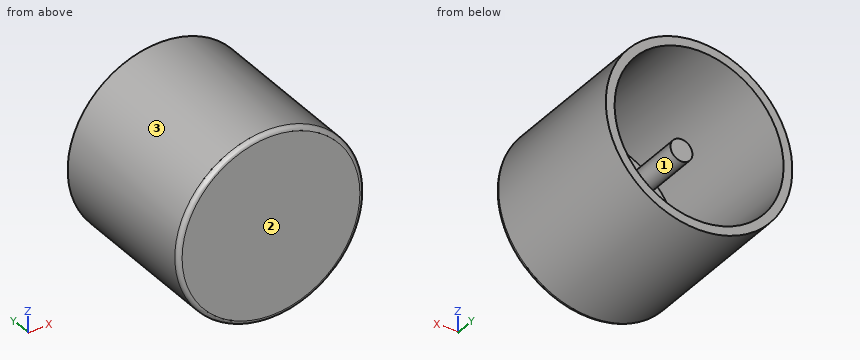
```python
from build123d import *

# Parameters (mm, degrees)
SKETCH1_R           = 53.975
BOSS_EXTRUDE1_DEPTH = 95.25
SHELL1_T            = -5.08
SKETCH2_R           = 6.35
BOSS_EXTRUDE2_DEPTH = 74.93
FILLET1_R           = 2.54


with BuildPart() as part:
    # Sketch1 → Boss-Extrude1 (new body)
    with BuildSketch(Plane(origin=(0, 0, 0), x_dir=(1, 0, 0), z_dir=(0, 1, 0))):
        with Locations(Location((0, 0, 0), (0, 0, 270))):
            Circle(SKETCH1_R)
    extrude(amount=BOSS_EXTRUDE1_DEPTH)

    # Shell1
    shell1_openings = [part.faces().sort_by_distance(p)[0] for p in [
        (0, 95.25, 0),
    ]]
    offset(amount=SHELL1_T, openings=shell1_openings, kind=Kind.INTERSECTION)

    # Sketch2 → Boss-Extrude2 (add)
    with BuildSketch(Plane(origin=(0, 5.08, 0), x_dir=(1, 0, 0), z_dir=(0, 1, 0))):
        with Locations(Location((0, 0, 0), (0, 0, 270))):
            Circle(SKETCH2_R)
    extrude(amount=BOSS_EXTRUDE2_DEPTH)

    # Fillet1
    fillet1_edges = [part.edges().sort_by_distance(p)[0] for p in [
        (0, 0, -53.975),
    ]]
    fillet(fillet1_edges, radius=FILLET1_R)


solid = part.part
```
Model file for the job. Use its own axes, mm. Face numbers are marked on the shaded views. Give positions to 0.01 mm unless a question says otherwise; leave off trailing zeros. Write each loop counter-clockwise with the first axis right and the second up, starting at its lowest first coordinate (ties: lowest second). Pieces come first, ordered by that corner, then holes. Notation, with made-up numbers: M -16,38 L 13,38 A9 cw 13,48 Z; hole C 74,48 d5. An arc over 180 degrees is marked long. Use a Markdown table: item, result.
1) Cut at C-C (z = 0). List the corners of the cut face in (x, y) (3 decimals).
Responses:
| item | result |
|---|---|
| outline | M -53.975,2.54 A2.54 ccw -51.435,0 L 51.435,0 A2.54 ccw 53.975,2.54 L 53.975,95.25 L 48.895,95.25 L 48.895,5.08 L 6.35,5.08 L 6.35,80.01 L -6.35,80.01 L -6.35,5.08 L -48.895,5.08 L -48.895,95.25 L -53.975,95.25 Z |
2) Cut at A-A (y = 40). List the corners of the cut face in (x, z) (3 decimals).
Responses:
| item | result |
|---|---|
| outline | C 0,0 d107.95; C 0,0 d12.7; hole C 0,0 d97.79 |
3) Drill centre lines: line 1 (X direction, y = 67, z = 0) (3 decimals); line 2 (Z direction, x = 5.5, y = 73); line 3 (Y direction, x = 38.5, z = -4). Where is each one in solid material? Low to high. Write a range as from..to.
Responses:
| item | result |
|---|---|
| line 1 | x = -53.975..-48.895, -6.35..6.35, 48.895..53.975 |
| line 2 | z = -53.69..-48.58, -3.17..3.17, 48.58..53.69 |
| line 3 | y = 0..5.08 |
4) Cut at B-B (x = 0). List the corners of the cut face in (y, z) (3 decimals).
Responses:
| item | result |
|---|---|
| outline | M 0,-51.435 A2.54 ccw 2.54,-53.975 L 95.25,-53.975 L 95.25,-48.895 L 5.08,-48.895 L 5.08,-6.35 L 80.01,-6.35 L 80.01,6.35 L 5.08,6.35 L 5.08,48.895 L 95.25,48.895 L 95.25,53.975 L 2.54,53.975 A2.54 ccw 0,51.435 Z |
5) Pin check, flat tips, straight feed: pin 1 (1 mm diameter, centred on y = 13, z = -1, fed in from +X); pin 2 (5 mm diameter, centred on x = 29, y = 27, fed in from -Z); pin 3 (6.5 mm diameter, centred on x = 1.5, z = 3, fed in from +Y). Stop position of each tip, or through.
Responses:
| item | result |
|---|---|
| pin 1 | stops at x = 53.97 |
| pin 2 | stops at z = -47.02 |
| pin 3 | stops at y = 80.01 |
6) Pull direction Z, two halves, no side cores. Call the marked faces 1, 2 and 3: +Z half, -Z half, draft (parallel to the pull), parting line (faces both ways), or undercut.
Responses:
| item | result |
|---|---|
| face 1 | undercut |
| face 2 | draft |
| face 3 | parting line |
